```python
from build123d import *

# Parameters (mm, degrees)
SKETCH1_W           = 20.5
SKETCH1_H           = 12
BOSS_EXTRUDE2_DEPTH = 2
SKETCH2_R           = 1.475
BOSS_EXTRUDE3_DEPTH = 4
FILLET1_R           = 1.475
FILLET2_R           = 0.2
BOSS_EXTRUDE4_DEPTH = 1.8
SKETCH6_R           = 2.25
CUT_EXTRUDE1_DEPTH  = 36.14832579
SKETCH7_W           = 18.806014856
SKETCH7_H           = 6.487022836
CUT_EXTRUDE2_DEPTH  = 29.95592861
SKETCH14_R          = 3.55
CUT_EXTRUDE4_DEPTH  = 8
CUT_EXTRUDE5_START  = -6
CUT_EXTRUDE5_DEPTH  = 6
SKETCH15_W          = 0.4
SKETCH15_H          = 2.666666667
CUT_EXTRUDE6_DEPTH  = 31.764359276


# Read off the part's stored shape, not the designer's step: Revolve2
with BuildPart() as part:
    # Sketch1 → Boss-Extrude2 (new body)
    with BuildSketch(Plane(origin=(0, 0, 0), x_dir=(1, 0, 0), z_dir=(0, 1, 0))):
        Rectangle(SKETCH1_W, SKETCH1_H)
    extrude(amount=BOSS_EXTRUDE2_DEPTH)

    # Sketch2 → Boss-Extrude3 (add)
    with BuildSketch(Plane(origin=(0, 2, 0), x_dir=(1, 0, 0), z_dir=(0, 1, 0))):
        with Locations(Location((-7.25, 3, 0), (0, 0, 90))):
            Circle(SKETCH2_R)
        with Locations(Location((7.25, 3, 0), (0, 0, 90))):
            Circle(SKETCH2_R)
    extrude(amount=BOSS_EXTRUDE3_DEPTH)

    # Fillet1
    fillet1_edges = [part.edges().sort_by_distance(p)[0] for p in [
        (-7.25, 6, -1.525),
        (7.25, 6, -1.525),
    ]]
    fillet(fillet1_edges, radius=FILLET1_R)

    # Fillet2
    fillet2_edges = [part.edges().sort_by_distance(p)[0] for p in [
        (-10.25, 2, 0),
        (0, 2, 6),
        (-7.25, 2, -1.525),
        (7.25, 2, -1.525),
        (10.25, 2, 0),
        (0, 2, -6),
    ]]
    fillet(fillet2_edges, radius=FILLET2_R)

    # Sketch3 → Boss-Extrude4 (add)
    with BuildSketch(Plane.XZ):
        with BuildLine():
            Line((10.25, -6), (24.517982167, -3.939264487))
            ThreePointArc((24.517982167, -3.939264487), (27.388306837, 0), (24.517982167, 3.939264487))
            Line((24.517982167, 3.939264487), (10.25, 6))
            Line((10.25, 6), (10.25, 0))
            Line((10.25, 0), (10.25, -6))
        make_face()
    boss_extrude4 = extrude(amount=-BOSS_EXTRUDE4_DEPTH)

    # Mirror1: Boss-Extrude4 across plane
    add(boss_extrude4.mirror(Plane(origin=(0, 0, 0), x_dir=(0, 0, 1), z_dir=(1, 0, 0))))

    # Revolve2 outline → Revolve2 (revolve)
    with BuildSketch(Plane(origin=(9.06, -9.06, 0), x_dir=(0.707106781186549, -0.707106781186546, 0), z_dir=(0, 0, 1))):
        Polygon((0, 14.085115852), (0, 7.082774875), (4.500000028, 7.082774875), (4.500000024, 17.312774899), (1.272340977, 14.085115852), align=None)
    revolve2 = revolve(axis=Axis((9.06, -9.06, 0), (0.707106781186546, 0.707106781186549, 0)))

    # Mirror2: Revolve2 across plane
    add(revolve2.mirror(Plane(origin=(0, 0, 0), x_dir=(0, 0, 1), z_dir=(1, 0, 0))))

    # Sketch6 → Cut-Extrude1 (cut, symmetric)
    with BuildSketch(Plane(origin=(5.008278144, 5.008278144, 0), x_dir=(0, 0, 1), z_dir=(-0.707106781186546, -0.707106781186549, 0))):
        with Locations(Location((0, -12.812774875, 0), (0, 0, 90))):
            Circle(SKETCH6_R)
    cut_extrude1 = extrude(amount=CUT_EXTRUDE1_DEPTH, both=True, mode=Mode.SUBTRACT)

    # Mirror3: Cut-Extrude1 across plane
    add(cut_extrude1.mirror(Plane(origin=(0, 0, 0), x_dir=(0, 0, 1), z_dir=(1, 0, 0))), mode=Mode.SUBTRACT)

    # Sketch7 → Cut-Extrude2 (cut, symmetric)
    with BuildSketch(Plane.XY):
        with Locations((19.653007428, 5.043511418)):
            Rectangle(SKETCH7_W, SKETCH7_H)
    cut_extrude2 = extrude(amount=CUT_EXTRUDE2_DEPTH, both=True, mode=Mode.SUBTRACT)

    # Mirror4: Cut-Extrude2 across plane
    add(cut_extrude2.mirror(Plane(origin=(0, 0, 0), x_dir=(0, 0, 1), z_dir=(1, 0, 0))), mode=Mode.SUBTRACT)

    # Sketch14 → Cut-Extrude4 (cut)
    with BuildSketch(Plane(origin=(-12.450990258, 12.450990258, 0), x_dir=(0, 0, -1), z_dir=(0.7071067811865438, -0.7071067811865512, 0))):
        with Locations(Location((0, -12.812774875, 0), (0, 0, 219.331248085))):
            Circle(SKETCH14_R)
    cut_extrude4 = extrude(amount=CUT_EXTRUDE4_DEPTH, mode=Mode.SUBTRACT)

    # Sketch14 → Cut-Extrude5 (cut)
    with BuildSketch(Plane(origin=(-12.450990258, 12.450990258, 0), x_dir=(0, 0, -1), z_dir=(0.7071067811865438, -0.7071067811865512, 0)).offset(CUT_EXTRUDE5_START)):
        with Locations(Location((0, -12.812774875, 0), (0, 0, 219.331248085))):
            Circle(SKETCH14_R)
    cut_extrude5 = extrude(amount=CUT_EXTRUDE5_DEPTH, mode=Mode.SUBTRACT)

    # Mirror5: Cut-Extrude4, Cut-Extrude5 across plane
    add(cut_extrude4.mirror(Plane(origin=(0, 0, 0), x_dir=(0, 0, 1), z_dir=(1, 0, 0))), mode=Mode.SUBTRACT)
    add(cut_extrude5.mirror(Plane(origin=(0, 0, 0), x_dir=(0, 0, 1), z_dir=(1, 0, 0))), mode=Mode.SUBTRACT)

    # Sketch15 → Cut-Extrude6 (cut, symmetric)
    with BuildSketch(Plane.XY.offset(6)):
        with Locations((-7.25, 4.666666667)):
            Rectangle(SKETCH15_W, SKETCH15_H)
    cut_extrude6 = extrude(amount=CUT_EXTRUDE6_DEPTH, both=True, mode=Mode.SUBTRACT)

    # Mirror6: Cut-Extrude6 across plane
    add(cut_extrude6.mirror(Plane(origin=(0, 0, 0), x_dir=(0, 0, 1), z_dir=(1, 0, 0))), mode=Mode.SUBTRACT)


solid = part.part
```
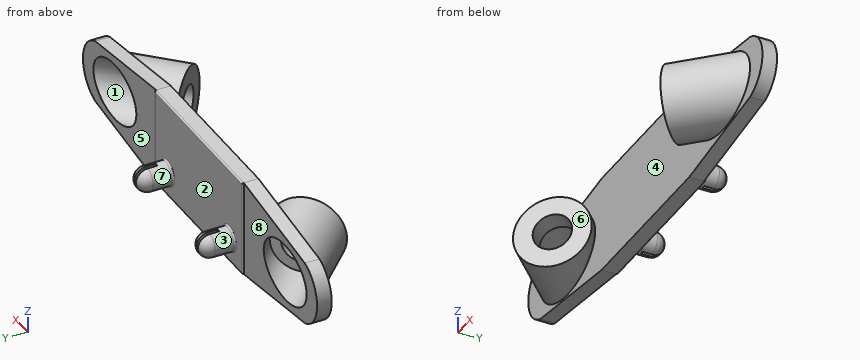
Model file for the job. Use its own axes, mm. Face numbers are marked on the shaded views. A direction names the side the tool comes from. Give positions to 0.01 mm unless a question says otherwise; leave off trailing zeros.
1) 3-axis set-ups, long thin cutter, end or side, ignore diameter. For the marked faces 4, 5, 6, 7 and 8: which of +Z, -Z, +X, -X, +Y, -Y reach the whole face in a straight line?
2) Saw through at B-B, the plane z = 1.5. Count the separate pieces of the cut face and the enclosed holes in it, then the cut area to 3 significant figures.
3) Mould opens along Z. For the marked faces 1, 2 and 3 say: +Z half, -Z half, draft (parallel to the pull), parting line (faces both ways), or undercut.
4) Pin check, flat tips, straight feed: pin 1 (3 mm diameter, centred on y = 4.5, z = -3, fed in from -X) (3 decimals); pin 2 (1 mm diameter, centred on y = -5.5, z = 0.5, fed in from +X); pin 3 (6 mm diameter, centred on x = 3, z = -0.5, fed in from +Y). Stop position of each tip, or through.
5) Wall check: probe 1 along X at (y, z) = (-2.75, -2.75); probe 2 along X at (y, z) = (-1, 0.75); probe 3 along Y at (x, z) = (9, 0.75). Give the ranges that are in metal, low to high.
Computed:
1. face 4: none
1. face 5: +Z, -Z, +X, +Y
1. face 6: +Z, -Z, -Y
1. face 7: +Y
1. face 8: +Z, -Z, -X, +Y
2. separate pieces: 3
2. enclosed holes: 0
2. area: 108 mm2
3. face 1: undercut
3. face 2: draft
3. face 3: parting line
4. pin 1: stops at x = -8.725
4. pin 2: stops at x = 19.45
4. pin 3: stops at y = 2
5. probe 1: x = -20.41 to -18.54, -16.34 to -12.77, 12.77 to 16.34, 18.54 to 20.41
5. probe 2: x = -23.39 to -22.03, -14.12 to -11.02, 11.02 to 14.12, 22.03 to 23.39
5. probe 3: y = 0 to 2
